Verification items for the finished model (mm, model axes). Face numbers are marked on the shaded views. Coordinates: 2 decimals unless noted, no trailing zeros. Write each loop counter-clockwise with the first axis right and the second up, starting at its lowest first coordinate (ties: lowest second). Pieces come first, ordered by that corner, then holes. Notation, with made-up numbers: M 11.25,28.25 L 23.25,28.25 A23 ccw 23.25,67.25 Z; hole C 46.25,-35 d1. An arc over 180 degrees is marked long. One line per item, written item: value.
```python
from build123d import *

# Parameters (mm, degrees)
SKETCH_1_R          = 15
SKETCH_1_R_2        = 3
EXTRUDE_1_DEPTH     = 2
SKETCH_2_R          = 0.95
CUT_EXTRUDE_1_REACH = 23.307
SKETCH_3_R          = 1.1
CUT_EXTRUDE_2_REACH = 28.571
SKETCH_5_R          = 3


with BuildPart() as part:
    # 草图1 → 凸台-拉伸1 (new body)
    with BuildSketch(Plane(origin=(0, 0, 0), x_dir=(1, 0, 0), z_dir=(0, 1, 0))):
        with Locations(Location((0, 0, 0), (0, 0, 270))):
            Circle(SKETCH_1_R)
        with Locations(Location((0, 0, 0), (0, 0, 270))):
            Circle(SKETCH_1_R_2, mode=Mode.SUBTRACT)
    extrude(amount=EXTRUDE_1_DEPTH)

    # 草图2 → 切除-旋转1 (revolve, cut)
    with BuildSketch(Plane.XY, mode=Mode.PRIVATE) as cut_revolve_1_sk:
        with Locations((9.05, 2)):
            Circle(SKETCH_2_R)
    revolve(cut_revolve_1_sk.sketch.rotate(Axis((0, 2, 0), (0, 1, 0)), 90), axis=Axis((0, 2, 0), (0, 1, 0)), mode=Mode.SUBTRACT)

    # 草图3 → 切除-拉伸1 (cut, up to next)
    with BuildSketch(Plane(origin=(0, 2, 0), x_dir=(1, 0, 0), z_dir=(0, 1, 0)), mode=Mode.PRIVATE) as cut_extrude_1_sk1:
        with Locations(Location((12.5, 0, 0), (0, 0, 270))):
            Circle(SKETCH_3_R)
    cut_extrude_1_tool1 = extrude(cut_extrude_1_sk1.sketch, amount=-CUT_EXTRUDE_1_REACH, mode=Mode.PRIVATE) & part.part
    # 草图3 → 切除-拉伸1 (cut, up to next)
    with BuildSketch(Plane(origin=(0, 2, 0), x_dir=(1, 0, 0), z_dir=(0, 1, 0)), mode=Mode.PRIVATE) as cut_extrude_1_sk2:
        with Locations(Location((0, -12.5, 0), (0, 0, 270))):
            Circle(SKETCH_3_R)
    cut_extrude_1_tool2 = extrude(cut_extrude_1_sk2.sketch, amount=-CUT_EXTRUDE_1_REACH, mode=Mode.PRIVATE) & part.part
    # 草图3 → 切除-拉伸1 (cut, up to next)
    with BuildSketch(Plane(origin=(0, 2, 0), x_dir=(1, 0, 0), z_dir=(0, 1, 0)), mode=Mode.PRIVATE) as cut_extrude_1_sk3:
        with Locations(Location((-12.5, 0, 0), (0, 0, 270))):
            Circle(SKETCH_3_R)
    cut_extrude_1_tool3 = extrude(cut_extrude_1_sk3.sketch, amount=-CUT_EXTRUDE_1_REACH, mode=Mode.PRIVATE) & part.part
    # 草图3 → 切除-拉伸1 (cut, up to next)
    with BuildSketch(Plane(origin=(0, 2, 0), x_dir=(1, 0, 0), z_dir=(0, 1, 0)), mode=Mode.PRIVATE) as cut_extrude_1_sk4:
        with Locations(Location((0, 12.5, 0), (0, 0, 270))):
            Circle(SKETCH_3_R)
    cut_extrude_1_tool4 = extrude(cut_extrude_1_sk4.sketch, amount=-CUT_EXTRUDE_1_REACH, mode=Mode.PRIVATE) & part.part
    add(cut_extrude_1_tool1.solids().sort_by_distance((12.5, 2, 0))[0], mode=Mode.SUBTRACT)
    add(cut_extrude_1_tool2.solids().sort_by_distance((0, 2, 12.5))[0], mode=Mode.SUBTRACT)
    add(cut_extrude_1_tool3.solids().sort_by_distance((-12.5, 2, 0))[0], mode=Mode.SUBTRACT)
    add(cut_extrude_1_tool4.solids().sort_by_distance((0, 2, -12.5))[0], mode=Mode.SUBTRACT)

    # 草图4 → 旋转1 (revolve)
    with BuildSketch(Plane(origin=(0, 0, 0), x_dir=(0, 0, -1), z_dir=(1, 0, 0))):
        Polygon((4, 0), (0, 0), (0, -16), (4, -16), (4.5, -11), (4, -11), (4.5, -6), (4, -6), (4.5, -1), (4, -1), align=None)
    revolve(axis=Axis((0, -16, 0), (0, 1, 0)))

    # 草图5 → 切除-拉伸2 (cut, up to next)
    with BuildSketch(Plane(origin=(0, 0, 0), x_dir=(1, 0, 0), z_dir=(0, 1, 0)), mode=Mode.PRIVATE) as cut_extrude_2_sk1:
        with Locations(Location((0, 0, 0), (0, 0, 270))):
            Circle(SKETCH_5_R)
    cut_extrude_2_tool1 = extrude(cut_extrude_2_sk1.sketch, amount=-CUT_EXTRUDE_2_REACH, mode=Mode.PRIVATE) & part.part
    add(cut_extrude_2_tool1.solids().sort_by_distance((0, 0, 0))[0], mode=Mode.SUBTRACT)


solid = part.part
```
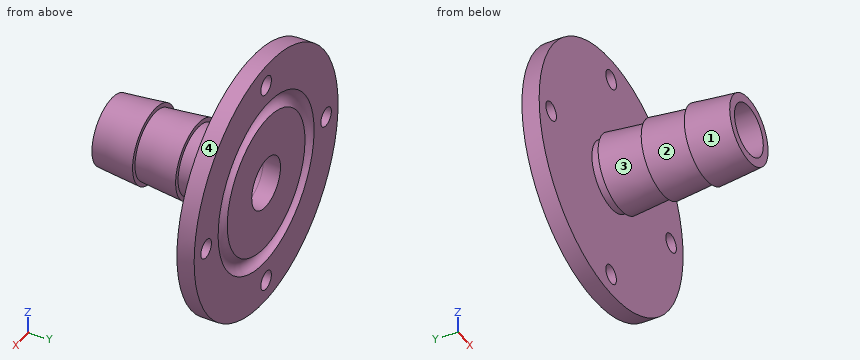
Item 1: Go/stop test with flat-tipped pins: P1, Ø10, axis at x = 9, z = 10, coming from the -Y side; P2, Ø10, axis at y = -11.5, z = 9, coming from the +X side; P3, Ø8, axis at x = 7, y = -3, coming from the -Z side. Record where each tip stops, or that it passes through.
The answers:
P1: stops at y = 0
P2: stops at x = 2.01
P3: stops at z = -14.35
Item 2: Cross-section at C-C, the plane z = 0. Give the number of separate pieces and of enclosed holes in the cut face, and give its area (3 significant figures).
The answers:
separate pieces: 4
enclosed holes: 0
area: 75.9 mm²
Item 3: Scan lines: line 1 (Z direction, x = 0.25, y = -9); line 2 (Y direction, x = 9.25, z = 11.5); line 3 (X direction, y = 0.8, z = 12.5). Record each from-to range of solid material in increasing order.
The answers:
line 1: z = -4.19 to -2.99, 2.99 to 4.19
line 2: y = 0 to 2
line 3: x = -8.29 to -1.1, 1.1 to 8.29
Item 4: Draft check along Y on the marked faces 1, 2, 3 and 4. Enter one of: released by +Y, released by -Y, zero draft, split by the parting line, or undercut.
The answers:
face 1: released by -Y
face 2: undercut
face 3: undercut
face 4: zero draft
Item 5: Cross-section at A-A, the plane x = -13. Enter the section's corners in (y, z), and give its area (3 significant figures).
The answers:
outline: M 0,-7.48 L 2,-7.48 L 2,-0.98 L 0,-0.98 Z; M 0,0.98 L 2,0.98 L 2,7.48 L 0,7.48 Z
area: 26.0 mm²
Item 6: Cross-section at B-B, the plane z = -12.5. Enter the section's corners in (x, y).
The answers:
outline: M -8.29,0 L -1.1,0 L -1.1,2 L -8.29,2 Z; M 1.1,0 L 8.29,0 L 8.29,2 L 1.1,2 Z
